Input: dimensioned drawing with shaded views. Units: mm. Origin: part minimum x, y, z. A direction names the side the tool comes from. Give positions to 0.01 mm unless a question says otherwise; leave off trailing zeros. Loops run counter-clockwise (first coordinate to the right, second up) from the corner with the lowest first, then second, coordinate; pieces in that order, holes last.
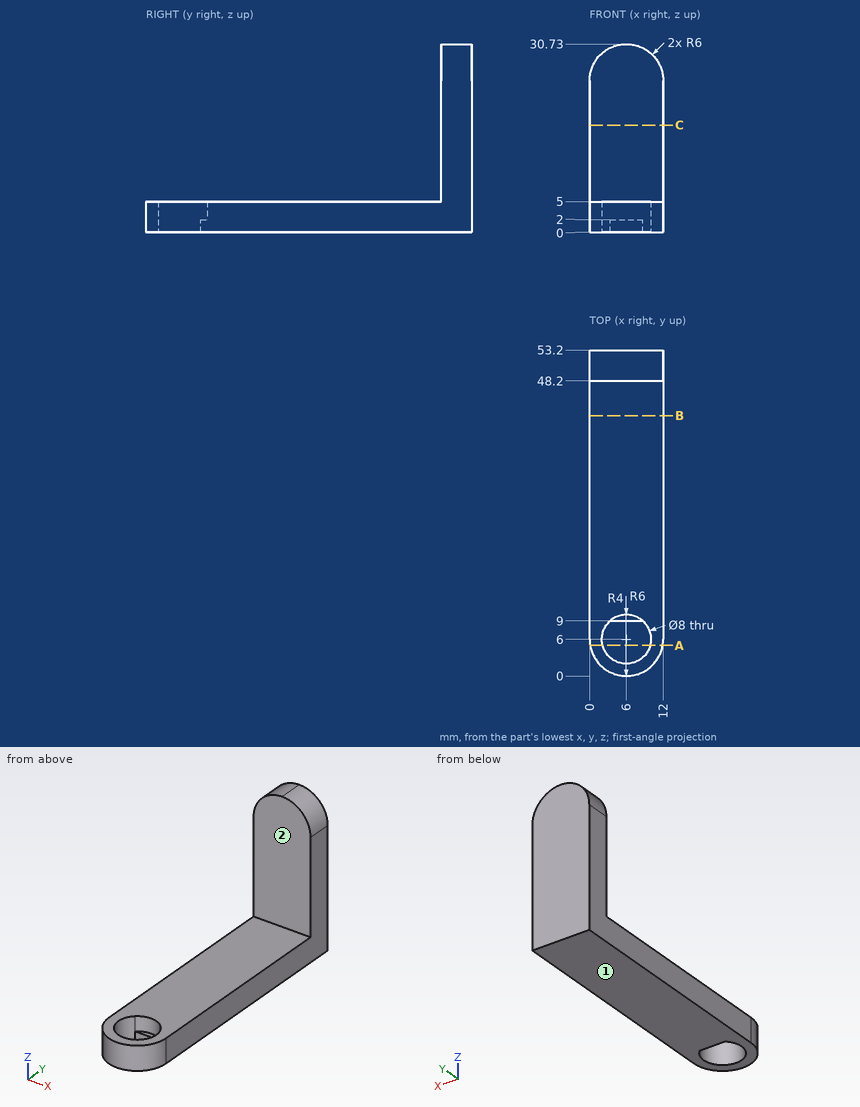
(1) Ray query, line 1 along X through (y, z) = (6, 2); line 2 along Z through (x, y) = (10, 27.5); line 3 along Y through (x, z) = (6.5, 11.5). Return the intervals inside material, ascending.
A:
line 1: x = 0 to 2, 10 to 12
line 2: z = 0 to 5
line 3: y = 48.2 to 53.2
(2) Reachability of the marked faces 1 and 2 from +Z, -Z, +X, -X, +Y, -Y: full face, straight path, thin tool, end or side. Return the list, or none.
A:
face 1: -Z, +X, -X, +Y, -Y
face 2: +Z, +X, -X, -Y
(3) Section B-B, the plane y = 42.5. Return the cut outline in (x, z).
A:
outline: (0, 0) - (12, 0) - (12, 5) - (0, 5) - close
(4) Section C-C, the plane z = 17.5. Return the cut outline in (x, y), then the cut area to 3 significant figures.
A:
outline: (0, 48.2) - (12, 48.2) - (12, 53.2) - (0, 53.2) - close
area: 60.0 mm2
(5) Section A-A, the plane y = 5. Return the cut outline in (x, z), then the cut area to 3 significant figures.
A:
outline: (0.08, 0) - (2.13, 0) - (2.13, 5) - (0.08, 5) - close; (9.87, 0) - (11.92, 0) - (11.92, 5) - (9.87, 5) - close
area: 20.4 mm2
(6) First-contact query: pin 1 (1.1 mm diameter, centred on x = 7, y = 9.5, fed in from +Z); pin 2 (3 mm diameter, centred on x = 7, z = 7.5, fed in from -Y); pin 3 (0.6 mm diameter, centred on x = 6.5, z = 1.5, fed in from -Y). Flat tips, straight axial feed; report the tip coordinate or a pass-through.
A:
pin 1: stops at z = 5
pin 2: stops at y = 48.2
pin 3: stops at y = 0
